from build123d import *

# Parameters (mm, degrees)
WYCI_GNI_CIE_PO_CIE_CE_CIENKA_CIAN_2_R   = 12.5
WYCI_GNI_CIE_PO_CIE_CE_CIENKA_CIAN_2_R_2 = 10


with BuildPart() as part:
    # Wyciągnięcie po ścieżce-Cienka ścianka1: sweep along a curve in space
    with BuildLine() as wyci_gni_cie_po_cie_ce_cienka_cianka1_path:
        Line((1151.551935215, -307.113467722, 173.439569165), (1129.696364798, -313.458624528, 165.695334052))
        Line((1151.551935215, -307.113467722, 173.439569165), (1185.156220245, -297.357398501, 185.346807417))
        ThreePointArc((1185.156220245, -297.357398501, 185.346807417), (1199.389809123, -294.346258299, 189.021890381), (1214.308973975, -293.326931287, 190.265974378))
        Line((1214.308973975, -293.326931287, 190.265974378), (1219.894910902, -293.326931287, 190.265974378))
        ThreePointArc((1235.622601719, -290.105182218, 190.265974378), (1227.922051201, -292.513217391, 190.265974378), (1219.894910902, -293.326931287, 190.265974378))
        Line((1235.622601719, -290.105182218, 190.265974378), (1265.932911584, -277.143413509, 190.265974378))
        ThreePointArc((1265.932911584, -277.143413509, 190.265974378), (1283.797363065, -269.747937613, 193.458288824), (1299.932584526, -263.553914321, 202.694698616))
        Line((1299.932584526, -263.553914321, 202.694698616), (1372.472988989, -237.060176471, 261.924171563))
        ThreePointArc((1372.472988989, -237.060176471, 261.924171563), (1382.771973534, -232.278738725, 272.935146818), (1389.58101162, -226.802870455, 286.119405336))
        Line((1389.58101162, -226.802870455, 286.119405336), (1403.276379011, -210.822780416, 325.305785456))
        ThreePointArc((1469.875752261, -192.528815146, 370.166250897), (1428.697459915, -197.586110339, 357.764750572), (1403.276379011, -210.822780416, 325.305785456))
    # Wyci_gni_cie po _cie_ce-Cienka _cian 2 (on start of the path) → Wyciągnięcie po ścieżce-Cienka ścianka1 (sweep)
    with BuildSketch(Plane(origin=(1469.875752261, -192.528815146, 370.166250897), x_dir=(0, 0, -1), z_dir=(-1, 0, 0))):
        Circle(WYCI_GNI_CIE_PO_CIE_CE_CIENKA_CIAN_2_R)
        Circle(WYCI_GNI_CIE_PO_CIE_CE_CIENKA_CIAN_2_R_2, mode=Mode.SUBTRACT)
    sweep(path=wyci_gni_cie_po_cie_ce_cienka_cianka1_path.line)


solid = part.part
Check sheet for the modelled part. Datum: model origin and axes. Units: mm. A direction names the side the tool comes from. Round coordinates to 2 decimals unless told otherwise and drop trailing zeros. One line per item, written item: value. Start each with the question number.
1. Scan lines: line 1 along Y through (x, z) = (1282, 186.5); line 2 along Y through (x, z) = (1353.5, 253.5); line 3 along Z through (x, y) = (1286, -263). Record each from-to range of solid material in increasing order.
2. Gauge pin test, flat ends, axial feed: P1, Ø2, axis at x = 1223.5, y = -284, coming from the -Z side; P2, Ø8, axis at x = 1373, y = -241.5, coming from the -Z side; P3, Ø8, axis at x = 1276, z = 203.5, coming from the +Y side. Record the tip position at first contact, or that the pin passes through.
3. Access from +Z, -Z, +X, -X, +Y, -Y to the whole of each face (thin tool, end or side, straight path). Record for faces 4 (the cylindrical face through (1217.063, -297.747, 181.296)), 5 (the flat face through (1132.225, -323.339, 166.653)).
4. Release check for a two-part mould opening along Y. For faces 1 (the cylindrical face through (1254.164, -292.13, 186.235)), 2 (the cylindrical face through (1217.06, -283.24, 182.88)), 3 (the flat face through (1469.876, -201, 376)) record: released by +Y, released by -Y, zero draft, split by the parting line, or undercut.
Results found:
1. line 1: -282.83 to -279.64, -262.68 to -259.52
1. line 2: -254.4 to -251.42, -234.03 to -231.05
1. line 3: 183.13 to 186.18, 204.45 to 207.7
2. P1: z = 180.76
2. P2: z = 242.95
2. P3: y = -260.75
3. face 4: none
3. face 5: -Z, -X, -Y
4. face 1: undercut
4. face 2: split by the parting line
4. face 3: zero draft
